```python
from build123d import *

# Parameters (mm, degrees)
SKETCH3_W           = 14
SKETCH3_H           = 8
BOSS_EXTRUDE2_DEPTH = 1.75


with BuildPart() as part:
    # Sketch2 → Revolve2 (revolve)
    with BuildSketch(Plane(origin=(0, 0, 0), x_dir=(0, 0, -1), z_dir=(1, 0, 0))):
        Polygon((34, 200), (42.5, 170), (42.5, 20), (42.5, 10), (42.5, 6), (34, 6), align=None)
    revolve(axis=Axis((0, 6, -34), (0, 1, 0)))

    # Sketch3 → Boss-Extrude2 (add, symmetric)
    with BuildSketch(Plane(origin=(0, 0, 0), x_dir=(0, 0, -1), z_dir=(1, 0, 0))):
        with Locations((27, 141)):
            Rectangle(SKETCH3_W, SKETCH3_H)
        with Locations((27, 51)):
            Rectangle(SKETCH3_W, SKETCH3_H)
    extrude(amount=BOSS_EXTRUDE2_DEPTH, both=True)


solid = part.part
```
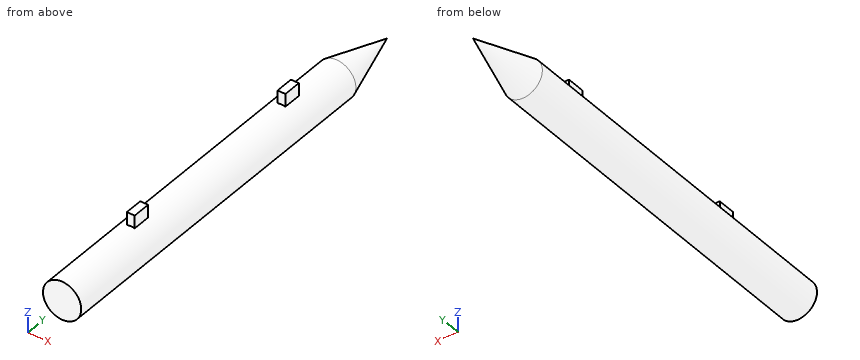
Check sheet for the modelled part. Datum: model origin and axes. Units: mm. Coordinates: 2 decimals unless noted, no trailing zeros. Order: outer loops, then holes, each group sorted by start corner. A loop starts at its lowest first (then second) coordinate and runs counter-clockwise, first axis right, second up. Notation, with made-up numbers: (36.5, -16.75) -> (55.5, -16.75) arc R12 ccw to (55.5, 5.25) -> close; hole circle Ø7 at (66, 44). An arc over 180 degrees is marked (long way). Write item = value, one per line. Start each with the question number.
1) Material ranges on L1, parallel to Y at x = 0, z = -21; L2, parallel to X at y = 52, z = -25.5; L3, parallel to Z at x = -4.25, y = 167.5, recorded low to high.
2) Cross-section at A-A (y = 142). Enter the section's corners in (x, z).
3) Go/stop test with flat-tipped pins: P1, Ø1.1, axis at x = -0.5, z = -22, coming from the -Y side; P2, Ø1.7, axis at y = 53, z = -21.5, coming from the -X side; P3, Ø4, axis at y = 67.5, z = -31, coming from the +X side; P4, Ø10, axis at x = 4, y = 136, coming from the +Z side. Record where each tip stops, or that it passes through.
4) Cross-section at B-B (y = 91). Enter the section's corners in (x, z).
Ans:
q1.L1 = 47 to 55, 137 to 145
q1.L2 = -1.75 to 1.75
q1.L3 = -41.36 to -26.64
q2.outline = (-1.75, -25.68) arc R8.5 ccw (long way) to (1.75, -25.68) -> (1.75, -20) -> (-1.75, -20) -> close
q3.P1 = 47
q3.P2 = -1.75
q3.P3 = 8.44
q3.P4 = -20
q4.outline = circle Ø17 at (0, -34)
